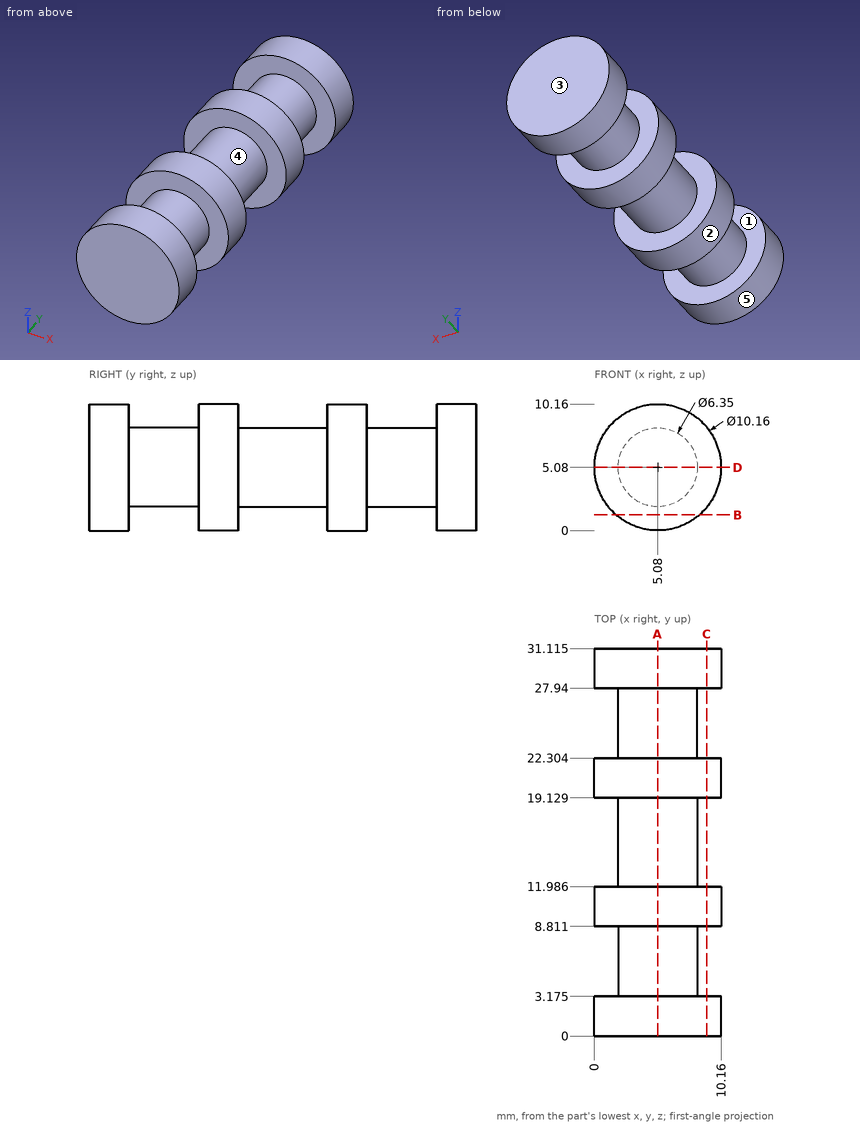
Drawing for the job (mm, zero at the part's lowest x, y, z). A direction names the side the tool comes from. Give positions to 0.01 mm unless a question says otherwise; leave off trailing zeros. Order: outer loops, then holes, each group sorted by start corner. A loop starts at its lowest first (then second) coordinate and runs counter-clockwise, first axis right, second up. Notation, with made-up numbers: M 42.25,65.25 L 91.25,65.25 A20 cw 91.25,84.25 Z; hole C 25.5,-17.5 d9. An arc over 180 degrees is marked long. Put each result on its own line as item: value. Start each with the question number.
(1) Flat gauge pins, fed straight in: pin 1 Ø4 at (y, z) = (11.5, 2) entering from +X; pin 2 Ø3 at (y, z) = (6, 5.5) entering from -X (3 decimals). Where does each tip first touch, or does it go through?
(2) Which spindle directions (+Z, -Z, +X, -X, +Y, -Y) get a long thin tool onto all of the face, cutting with end or side? Do the marked faces 1 and 2. Say none if no direction does.
(3) Saw through at A-A, the plane x = 5.08. Write the cut outline in (y, z) (1 decimal), then the cut area to 3 significant figures.
(4) Saw through at C-C, the plane x = 9. Write the cut outline in (y, z) (1 decimal).
(5) Saw through at B-B, the plane z = 1.25. Write the cut outline in (x, y) (1 decimal).
(6) Saw through at D-D, the plane z = 5.08. Write the cut outline in (x, y) (1 decimal), then the cut area to 3 significant figures.
(7) Drill centre lines: line 1 along Y through (x, z) = (9.75, 5) (1 decimal); line 2 along X through (y, z) = (22, 8.75) (1 decimal); line 3 along X through (y, z) = (9, 5.5). Where is each one in solid material? Low to high.
(8) Mould opens along Y. For the marked faces 3, 4 and 5 say: +Y half, -Y half, draft (parallel to the pull), parting line (faces both ways), or undercut.
Check result:
1. pin 1: stops at x = 10.04
1. pin 2: stops at x = 1.905
2. face 1: none
2. face 2: +Y, -Y
3. outline: M 0,0 L 3.2,0 L 3.2,1.9 L 8.8,1.9 L 8.8,0 L 12,0 L 12,1.9 L 19.1,1.9 L 19.1,0 L 22.3,0 L 22.3,1.9 L 27.9,1.9 L 27.9,0 L 31.1,0 L 31.1,10.2 L 27.9,10.2 L 27.9,8.3 L 22.3,8.3 L 22.3,10.2 L 19.1,10.2 L 19.1,8.3 L 12,8.3 L 12,10.2 L 8.8,10.2 L 8.8,8.3 L 3.2,8.3 L 3.2,10.2 L 0,10.2 Z
3. area: 246 mm2
4. outline: M 0,1.8 L 3.2,1.8 L 3.2,8.3 L 0,8.3 Z; M 8.8,1.8 L 12,1.8 L 12,8.3 L 8.8,8.3 Z; M 19.1,1.8 L 22.3,1.8 L 22.3,8.3 L 19.1,8.3 Z; M 27.9,1.8 L 31.1,1.8 L 31.1,8.3 L 27.9,8.3 Z
5. outline: M 1.7,0 L 8.4,0 L 8.4,3.2 L 1.7,3.2 Z; M 1.7,8.8 L 8.4,8.8 L 8.4,12 L 1.7,12 Z; M 1.7,19.1 L 8.4,19.1 L 8.4,22.3 L 1.7,22.3 Z; M 1.7,27.9 L 8.4,27.9 L 8.4,31.1 L 1.7,31.1 Z
6. outline: M 0,0 L 10.2,0 L 10.2,3.2 L 8.3,3.2 L 8.3,8.8 L 10.2,8.8 L 10.2,12 L 8.3,12 L 8.3,19.1 L 10.2,19.1 L 10.2,22.3 L 8.3,22.3 L 8.3,27.9 L 10.2,27.9 L 10.2,31.1 L 0,31.1 L 0,27.9 L 1.9,27.9 L 1.9,22.3 L 0,22.3 L 0,19.1 L 1.9,19.1 L 1.9,12 L 0,12 L 0,8.8 L 1.9,8.8 L 1.9,3.2 L 0,3.2 Z
6. area: 246 mm2
7. line 1: y = 0 to 3.2, 8.8 to 12, 19.1 to 22.3, 27.9 to 31.1
7. line 2: x = 1.6 to 8.6
7. line 3: x = 0.02 to 10.14
8. face 3: +Y half
8. face 4: undercut
8. face 5: draft
